Can you work these out from the model? Positions are in its coordinate system, mm. A direction names the side the tool comes from. Round coordinates to 2 decimals unless told otherwise and drop trailing zeros. Loops run counter-clockwise (first coordinate to the right, second up) from the corner with the lowest first, then second, coordinate; pieces in that order, holes last. Notation, with made-up numbers: (46, -18) -> (98, -18) arc R10 cw to (98, -12) -> close; hole circle Ø11 at (79, 28). An arc over 180 degrees is marked (long way). Write item = value, one per line.
from build123d import *

# Parameters (mm, degrees)
CREATE_INTERNAL_GEOMETRY_DEPTH = 38
CUT_SHACKLE_HOLE_DEPTH         = 83.24962006
CAP_TOP_END_DEPTH              = 4
ROUND_CORNERS_R                = 10
UNNECESSARY_CHAMFERS_SIZE      = 1


with BuildPart() as part:
    # Sketch2 → Create internal geometry (new body)
    with BuildSketch(Plane(origin=(0, 0, 0), x_dir=(1, 0, 0), z_dir=(0, 1, 0))):
        Polygon((36.236067977, 20), (-7.763932023, 42), (-25, 42), (-25, 27), (4.236067977, 27), (26.236067977, 16), (57, 16), (57, 6), (26.155256109, 6), (4.155256109, -1), (0, -1), (0, -5), (4.776280544, -5), (26.776280544, 2), (61, 2), (61, 20), align=None)
    extrude(amount=CREATE_INTERNAL_GEOMETRY_DEPTH)

    # Sketch4 → Cut shackle hole (cut, through all)
    with BuildSketch(Plane.XY.offset(-2)):
        with BuildLine():
            Line((49.5, 27), (49.5, 11))
            ThreePointArc((49.5, 11), (45.5, 7), (41.5, 11))
            Line((41.5, 11), (41.5, 27))
            ThreePointArc((41.5, 27), (45.5, 31), (49.5, 27))
        make_face()
    extrude(amount=-CUT_SHACKLE_HOLE_DEPTH, mode=Mode.SUBTRACT)

    # Sketch3 → Cap top end (add)
    with BuildSketch(Plane(origin=(0, 38, 0), x_dir=(1, 0, 0), z_dir=(0, 1, 0))):
        with BuildLine():
            Line((-25, 27), (2.155256109, 27))
            ThreePointArc((2.155256109, 27), (3.569469671, 26.414213562), (4.155256109, 25))
            Line((4.155256109, 25), (4.155256109, 1))
            ThreePointArc((4.155256109, 1), (3.569469671, -0.414213562), (2.155256109, -1))
            Line((2.155256109, -1), (0, -1))
            Line((0, -1), (0, -5))
            Line((0, -5), (4.776280544, -5))
            Line((4.776280544, -5), (26.776280544, 2))
            Line((26.776280544, 2), (61, 2))
            Line((61, 2), (61, 20))
            Line((61, 20), (36.236067977, 20))
            Line((36.236067977, 20), (-7.763932023, 42))
            Line((-7.763932023, 42), (-25, 42))
            Line((-25, 42), (-25, 27))
        make_face()
    cap_top_end = extrude(amount=CAP_TOP_END_DEPTH)

    # Mirror top cap to bottom: Cap top end across plane
    add(cap_top_end.mirror(Plane.ZX.offset(19)))

    # Round corners
    round_corners_edges = [part.edges().sort_by_distance(p)[0] for p in [
        (61, -4, -11),
        (57, 0, -11),
        (57, 38, -11),
        (61, 42, -11),
    ]]
    fillet(round_corners_edges, radius=ROUND_CORNERS_R)

    # Unnecessary chamfers
    unnecessary_chamfers_edges = [part.edges().sort_by_distance(p)[0] for p in [
        (-25, -4, -34.5),
        (-16.381966011, -4, -42),
        (14.236067977, -4, -31),
        (38.888140272, -4, -2),
        (15.776280544, -4, 1.5),
        (2.388140272, -4, 5),
        (0, -4, 3),
        (1.077628054, -4, 1),
        (3.569469671, -4, 0.414213562),
        (4.155256109, -4, -13),
        (3.569469671, -4, -26.414213562),
        (-11.422371946, -4, -27),
        (43.618033989, 42, -20),
        (61, 19, -20),
        (43.618033989, -4, -20),
        (58.071067812, -1.071067812, -20),
        (58.071067812, 39.071067812, -20),
        (61, 19, -2),
        (58.071067812, -1.071067812, -2),
        (58.071067812, 39.071067812, -2),
        (0, 19, 1),
        (-25, 19, -27),
        (-25, 19, -42),
        (0, 19, 5),
        (45.5, 31, -20),
        (49.5, 19, -20),
        (45.5, 7, -20),
        (41.5, 19, -20),
        (45.5, 31, -2),
        (41.5, 19, -2),
        (45.5, 7, -2),
        (49.5, 19, -2),
        (-25, 42, -34.5),
        (-11.422371946, 42, -27),
        (3.569469671, 42, -26.414213562),
        (4.155256109, 42, -13),
        (3.569469671, 42, 0.414213562),
        (1.077628054, 42, 1),
        (0, 42, 3),
        (2.388140272, 42, 5),
        (15.776280544, 42, 1.5),
        (38.888140272, 42, -2),
        (14.236067977, 42, -31),
        (-16.381966011, 42, -42),
    ]]
    chamfer(unnecessary_chamfers_edges, length=UNNECESSARY_CHAMFERS_SIZE)


solid = part.part
1. Suppose I cut it at A-A, the plane y = 16. Count the separate pieces of the cut face and the enclosed holes in it, and give its area (3 significant figures).
Entries:
separate_pieces = 3
enclosed_holes = 0
area = 984 mm²
2. Suppose I cut it at B-B, the plane x = 16. List the corners of the cut face in (y, z) for me, and give its area (3 significant figures).
Entries:
outline = (-4, -29) -> (-3, -30.12) -> (41, -30.12) -> (42, -29) -> (42, 0.38) -> (41, 1.43) -> (-3, 1.43) -> (-4, 0.38) -> close; hole (0, -21.12) -> (38, -21.12) -> (38, -2.77) -> (0, -2.77) -> close
area = 752 mm²
3. I need wall thicknesses on line 1 (Y direction, x = 36, z = -13.5); line 2 (Z direction, x = 56, y = 20); line 3 (Z direction, x = 10.5, y = 1). Which ranges of each line are inside material? Lowest first, please. Write a range as [from, to].
Entries:
line_1 = [-4, 0], [38, 42]
line_2 = [-20, -16], [-6, -2]
line_3 = [-32.87, -23.87], [-1.02, 3.18]
4. For faces 1 (the flat face through (51, 19, -20)), 2 (the flat face through (15.08, 18.73, -21.58)), 3 (the conical face through (3.82, 41.38, -26.7)), 4 (the conical face through (45.6, 6.8, -2.8)), 5 (the cylindrical face through (45.4, 31, -17.5)), which set-ups out of +Z, -Z, +X, -X, +Y, -Y let a thin tool reach every point of the face, with its end or its side?
Entries:
face_1 = -Z, +X, +Y, -Y
face_2 = -X
face_3 = -X, +Y
face_4 = +Z
face_5 = +Z, -Z
5. Suppose I cut it at D-D, the plane x = 28. List the corners of the cut face in (y, z) for me, and give its area (3 significant figures).
Entries:
outline = (-4, -23) -> (-3, -24.12) -> (41, -24.12) -> (42, -23) -> (42, -3) -> (41, -2) -> (-3, -2) -> (-4, -3) -> close; hole (0, -16) -> (38, -16) -> (38, -6) -> (0, -6) -> close
area = 635 mm²
6. I'm going to push flat-ended pins straight in: pin 1 (1 mm diameter, centred on y = 16, z = 3.5, fed in from -X); pin 2 (1.5 mm diameter, centred on y = 18.5, z = -17.5, fed in from -X); pin 3 (1 mm diameter, centred on x = 35, y = 9, fed in from +Z); pin 4 (12 mm diameter, centred on x = 33.5, z = -32.5, fed in from +Y). Where does each tip first touch, or does it pass through?
Entries:
pin_1 = 0
pin_2 = 21.74
pin_3 = -2
pin_4 = through
7. Suppose I cut it at C-C, the plane z = -30. List the corners of the cut face in (x, y) for me.
Entries:
outline = (-25, -3) -> (-24, -4) -> (14, -4) -> (16.24, -3) -> (16.24, 41) -> (14, 42) -> (-24, 42) -> (-25, 41) -> close
8. We'd pull the mould along Z, two halves only. Please class faces 6 (the cylindrical face through (54.15, 3.01, -10.93)), 7 (the flat face through (39, 19, -2)), 8 (the flat face through (14.431, 41.493, -30.352)): released by +Z, released by -Z, zero draft, split by the parting line, or undercut.
Entries:
face_6 = undercut
face_7 = released by +Z
face_8 = released by -Z
